Geometry check sheet. Reference: the model listing, model coordinates, mm. Face numbers are marked on the shaded views. Give positions to 0.01 mm unless a question says otherwise; leave off trailing zeros. Write each loop counter-clockwise with the first axis right and the second up, starting at its lowest first coordinate (ties: lowest second). Pieces come first, ordered by that corner, then holes.
(1) Depth check by flat-ended pin: P1, Ø1.5, axis at x = 56, y = -5.5, coming from the -Z side; P2, Ø1.2, axis at x = 47.5, z = -16, coming from the +Y side; P3, Ø2, axis at x = -34, y = -3, coming from the +Z side. Enter the tip coordinate at first touch or a pass-through.
(2) Thickness scan on line 1 along Z through (x, y) = (93, -5); line 2 along Y through (x, z) = (-34.5, 2); line 3 along Y through (x, z) = (120, -14). Record the ranges inside material, lowest first.
(3) Mould release check, pull along Z, two halves, no side actions. Record for the marked faces 1 and 2: +Z half, -Z half, draft (parallel to the pull), parting line (faces both ways), or undercut.
(4) Cross-section at A-A (y = -4.25). Record the boundary of the cut face in (x, z), and give its area (3 significant figures).
(5) Cross-section at C-C (z = 0.5). Record the boundary of the cut face in (x, y).
(6) Cross-section at B-B (x = 5.5). Record the boundary of the cut face in (y, z), and give its area (3 significant figures).
```python
from build123d import *

# Parameters (mm, degrees)
PAD005_DEPTH = 139
FILLET_R     = 1
FILLET001_R  = 1


with BuildPart() as part:
    # Sketch005 → Pad005 (new body, symmetric)
    with BuildSketch(Plane.YZ):
        Polygon((0, 13.5), (0, -13.5), (-6.5, -13.5), (-6.5, -17.5), (-7.5, -17.5), (-7.5, -12.5), (-1, -12.5), (-1, 12.5), (-7.5, 12.5), (-7.5, 17.5), (-6.5, 17.5), (-6.5, 13.5), align=None)
    extrude(amount=PAD005_DEPTH, both=True)

    # Fillet
    fillet_edges = [part.edges().sort_by_distance(p)[0] for p in [
        (0, -7.5, -12.5),
    ]]
    fillet(fillet_edges, radius=FILLET_R)

    # Fillet001
    fillet001_edges = [part.edges().sort_by_distance(p)[0] for p in [
        (0, -7.5, 12.5),
    ]]
    fillet(fillet001_edges, radius=FILLET001_R)


solid = part.part
```
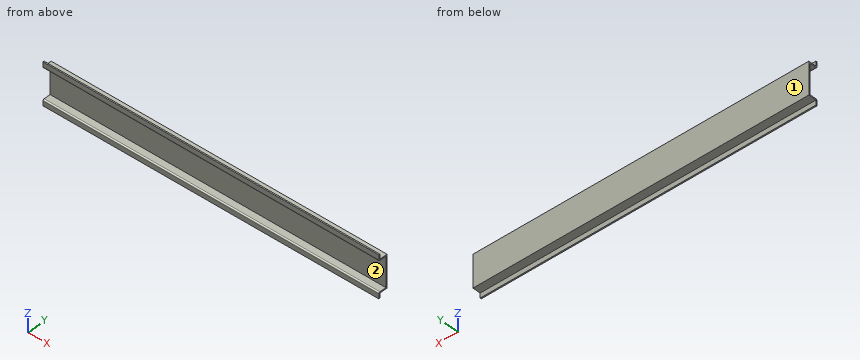
Reply:
1. P1: stops at z = -13.5
1. P2: stops at y = -6.5
1. P3: stops at z = 13.5
2. line 1: z = -13.5 to -12.5, 12.5 to 13.5
2. line 2: y = -1 to 0
2. line 3: y = -7.5 to -6.5
3. face 1: draft
3. face 2: undercut
4. outline: (-139, -13.5) - (139, -13.5) - (139, -12.5) - (-139, -12.5) - close; (-139, 12.5) - (139, 12.5) - (139, 13.5) - (-139, 13.5) - close
4. area: 556 mm2
5. outline: (-139, -1) - (139, -1) - (139, 0) - (-139, 0) - close
6. outline: (-7.5, -17.5) - (-6.5, -17.5) - (-6.5, -13.5) - (0, -13.5) - (0, 13.5) - (-6.5, 13.5) - (-6.5, 17.5) - (-7.5, 17.5) - (-7.5, 13.5) arc R1 ccw to (-6.5, 12.5) - (-1, 12.5) - (-1, -12.5) - (-6.5, -12.5) arc R1 ccw to (-7.5, -13.5) - close
6. area: 47.6 mm2
